Part model, mm, in its own coordinate system. Face numbers are marked on the shaded views. A direction names the side the tool comes from. Round coordinates to 2 decimals unless told otherwise and drop trailing zeros. Order: outer loops, then holes, each group sorted by start corner. A loop starts at its lowest first (then second) coordinate and runs counter-clockwise, first axis right, second up. Notation, with made-up numbers: (36, 59) -> (94, 59) arc R26 cw to (94, 91) -> close; hole circle Ø4 at (36, 0). An arc over 180 degrees is marked (long way). Use CSV: the item, a comma, the result in double quotes.
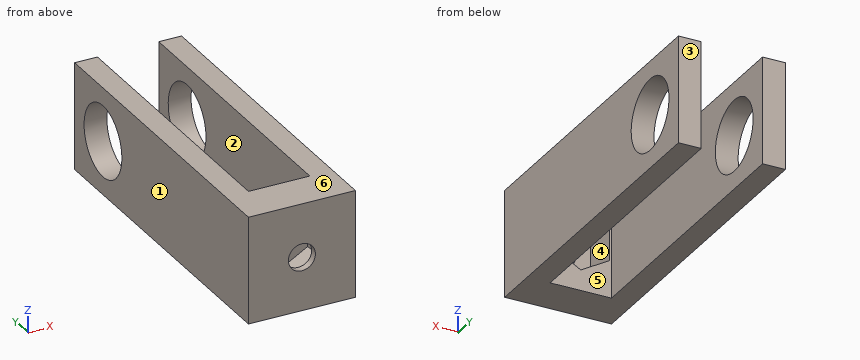
Autodesk Inventor part; units mm, degrees
ref_plane "YZ Plane" through (0, 0, 0) normal (1, 0, 0) x (0, 1, 0)
ref_plane "XZ Plane" through (0, 0, 0) normal (0, 1, 0) x (-1, 0, 0)
ref_plane "XY Plane" through (0, 0, 0) normal (0, 0, 1) x (1, 0, 0)
sketch "Sketch1" plane through (0, 0, 0) normal (0, 1, 0) x (-1, 0, 0)
  line L0 (0, 0) -> (19.05, 0)
  line L1 (19.05, 0) -> (19.05, -19.05)
  line L2 (19.05, -19.05) -> (0, -19.05)
  line L3 (0, -19.05) -> (0, 0)
  dimension "d0" = 19.05
  dimension "d1" = 19.05
extrude "Extrusion1" add sketch "Sketch1" along normal blind 7.62
sketch "Sketch2" plane through (0, 7.62, 0) normal (0, 1, 0) x (1, 0, 0)
  line L0 (-9.525, 3.6591) -> (-14.605, 6.5921)
  line L1 (-14.605, 6.5921) -> (-14.605, 12.4579)
  line L2 (-14.605, 12.4579) -> (-9.525, 15.3909)
  line L3 (-9.525, 15.3909) -> (-4.445, 12.4579)
  line L4 (-4.445, 12.4579) -> (-4.445, 6.5921)
  line L5 (-4.445, 6.5921) -> (-9.525, 3.6591)
  line L6 (0, 19.05) -> (-19.05, 19.05)
  line L7 (0, 0) -> (0, 19.05)
  point P0 (-9.525, 9.525)
  dimension "d4" = 10.16
  dimension "d5" = 9.525
  dimension "d6" = 9.525
extrude "Extrusion2" cut sketch "Sketch2" against normal blind 6.35
sketch "Sketch3" plane through (0, 1.27, 0) normal (0, 1, 0) x (1, 0, 0)
  circle A0 centre (-9.525, 9.525) radius 2.413
  line L0 (-14.605, 12.4579) -> (-9.525, 15.3909)
  line L1 (-9.525, 3.6591) -> (-14.605, 6.5921)
  point P0 (0, 0)
  dimension "d9" = 4.826
  dimension "d10" = 5.08
  dimension "d11" = 5.08
extrude "Extrusion3" cut sketch "Sketch3" against normal blind 12.7
sketch "Sketch4" plane through (0, 7.62, 0) normal (0, 1, 0) x (1, 0, 0)
  line L0 (0, 19.05) -> (-19.05, 19.05)
  line L1 (-19.05, 19.05) -> (-14.986, 19.05)
  line L2 (-14.986, 19.05) -> (-14.986, 0)
  line L3 (-14.986, 0) -> (-19.05, 0)
  line L4 (-19.05, 0) -> (-19.05, 19.05)
  line L5 (0, 19.05) -> (-4.064, 19.05)
  line L6 (-4.064, 19.05) -> (-4.064, 0)
  line L7 (-4.064, 0) -> (0, 0)
  line L8 (0, 0) -> (0, 19.05)
  line L9 (-19.05, 0) -> (0, 0)
  dimension "d14" = 4.064
  dimension "d15" = 4.064
extrude "Extrusion4" add sketch "Sketch4" along normal blind 50.8 contours L8 L7 L6 L0 | L2 L3 L4 L0
sketch "Sketch5" plane through (-19.05, 0, -19.05) normal (-1, 0, 0) x (0, 0, 1)
  circle A0 centre (9.525, 48.895) radius 6.35
  line L0 (19.05, 0) -> (19.05, 58.42)
  line L1 (0, 58.42) -> (19.05, 58.42)
  dimension "d18" = 12.7
  dimension "d19" = 9.525
  dimension "d20" = 9.525
extrude "Extrusion5" cut sketch "Sketch5" against normal blind 19.05
properties part number "silider shaft" material "ABS Plastic"
(1) Which spindle directions (+Z, -Z, +X, -X, +Y, -Y) get a long thin tool onto all of the face, cutting with end or side? Do the marked faces 4, 5 and 6. Say none if no direction does.
Reply:
face 4,"+Y"
face 5,"+Z, -Z, +Y"
face 6,"+Z, +X, -X, +Y, -Y"
(2) Drop flat-ended pins along their axis: P1, Ø3.5, axis at x = -8, z = -7.5, coming from the +Y side; P2, Ø4, axis at x = -9.525, z = -9.525, coming from the -Y side; P3, Ø4, axis at x = -9, z = -4.5, coming from the +Y side. Give the stop position or say it passes through.
Reply:
P1,"y = 1.27"
P2,"through"
P3,"y = 7.62"
(3) Cut at D-D, the plane z = -14.5. Give the cut face in (x, y), then the cut area to 3 significant figures.
Reply:
outline,"(-19.05, 0) -> (0, 0) -> (0, 44.95) -> (-4.06, 44.95) -> (-4.06, 7.62) -> (-7.98, 7.62) -> (-7.98, 1.27) -> (-11.07, 1.27) -> (-11.07, 7.62) -> (-14.99, 7.62) -> (-14.99, 44.95) -> (-19.05, 44.95) -> close; (-19.05, 52.84) -> (-14.99, 52.84) -> (-14.99, 58.42) -> (-19.05, 58.42) -> close; (-4.06, 52.84) -> (0, 52.84) -> (0, 58.42) -> (-4.06, 58.42) -> close"
area,"474 mm2"
(4) Cut at C-C, the plane z = -17.25. Give the cut face in (x, y).
Reply:
outline,"(-19.05, 0) -> (0, 0) -> (0, 58.42) -> (-4.06, 58.42) -> (-4.06, 7.62) -> (-14.99, 7.62) -> (-14.99, 58.42) -> (-19.05, 58.42) -> close"
(5) Cut at B-B, the plane x = -11. Give the cut face in (y, z).
Reply:
outline,"(0, -19.05) -> (7.62, -19.05) -> (7.62, -14.54) -> (1.27, -14.54) -> (1.27, -11.43) -> (0, -11.43) -> close; (0, -7.62) -> (1.27, -7.62) -> (1.27, -4.51) -> (7.62, -4.51) -> (7.62, 0) -> (0, 0) -> close"
(6) Pull direction X, two halves, no side cores. Call the marked faces 1, 2 and 3: released by +X, released by -X, zero draft, split by the parting line, or undercut.
Reply:
face 1,"released by -X"
face 2,"undercut"
face 3,"zero draft"
(7) Probe probe 1 along X at (y, z) = (36, -10); probe 2 along Y at (x, z) = (-5.25, -5.25); probe 3 along Y at (x, z) = (-11, -7.5). List the from-to ranges inside material, lowest first. Write a range as [from, to].
Reply:
probe 1,"[-19.05, -14.99], [-4.06, 0]"
probe 2,"[0, 7.62]"
probe 3,"[0, 1.27]"
(8) Cut at A-A, the plane y = 8.5. Give the cut face in (x, z).
Reply:
outline,"(-19.05, -19.05) -> (-14.99, -19.05) -> (-14.99, 0) -> (-19.05, 0) -> close; (-4.06, -19.05) -> (0, -19.05) -> (0, 0) -> (-4.06, 0) -> close"
